```python
from build123d import *

# Parameters (mm, degrees)
SKETCH2_R           = 2.5
BOSS_EXTRUDE1_DEPTH = 12
CUT_EXTRUDE1_DEPTH  = 2.2
CHAMFER1_SIZE       = 0.55
CHAMFER2_SIZE       = 0.35
CHAMFER2_SIZE2      = 0.6


with BuildPart() as part:
    # Sketch1 → Revolve1 (revolve)
    with BuildSketch(Plane.XY.offset(9.9)):
        with BuildLine():
            Line((2.4, 14.65), (2.4, 9.9))
            Line((2.4, 9.9), (5.15, 9.9))
            Line((5.15, 9.9), (5.15, 11.8))
            ThreePointArc((5.15, 11.8), (4.281848259, 13.427774941), (2.899999999, 14.65))
            Line((2.899999999, 14.65), (2.4, 14.65))
        make_face()
    revolve(axis=Axis((2.4, 9.9, 9.9), (1, 0, 0)))

    # Sketch2 → Boss-Extrude1 (add)
    with BuildSketch(Plane.ZY.offset(-2.4)):
        with Locations((9.9, 9.9)):
            Circle(SKETCH2_R)
    extrude(amount=BOSS_EXTRUDE1_DEPTH)

    # Sketch3 → Cut-Extrude1 (cut)
    with BuildSketch(Plane(origin=(5.15, 0, 0), x_dir=(0, 0, -1), z_dir=(1, 0, 0))):
        Polygon((-11.6320508, 9.9), (-10.766025397, 8.400000002), (-9.033974587, 8.400000002), (-8.167949184, 9.9), (-9.033974587, 11.399999998), (-10.766025397, 11.399999998), align=None)
    extrude(amount=-CUT_EXTRUDE1_DEPTH, mode=Mode.SUBTRACT)

    # Chamfer1
    chamfer1_edges = [part.edges().sort_by_distance(p)[0] for p in [
        (-9.6, 9.9, 7.4),
    ]]
    chamfer(chamfer1_edges, length=CHAMFER1_SIZE)

    # Chamfer2
    chamfer2_edges = [part.edges().sort_by_distance(p)[0] for p in [
        (2.4, 9.9, 7.4),
    ]]
    chamfer2_side = [part.faces().sort_by_distance(p)[0] for p in [
        (2.4, 5.284350289, 9.9),
    ]]
    chamfer(chamfer2_edges, length=CHAMFER2_SIZE, length2=CHAMFER2_SIZE2, reference=chamfer2_side[0])


solid = part.part
```
Source: CAD feature listing. Evaluate the final solid. Frame: model axes, mm. A direction names the side the tool comes from. Give positions to 0.01 mm unless a question says otherwise; leave off trailing zeros. Loops run counter-clockwise (first coordinate to the right, second up) from the corner with the lowest first, then second, coordinate; pieces in that order, holes last. Notation, with made-up numbers: (6, 67.25) -> (46, 67.25) arc R12 cw to (46, 73.25) -> close; hole circle Ø10 at (36.25, 73). An arc over 180 degrees is marked (long way). Put each result on its own line as item: value. Start each with the question number.
1) Draft query along Z for faces 4 (the face through (2.4, 9.8, 6.8)), 5 (the face through (4, 8.4, 10)), 6 (the face through (2.646, 14.288, 8.081)). Return one class per face: released by +Z, released by -Z, zero draft, split by the parting line, or undercut.
2) Material intervals for probe 1 along X at (y, z) = (11, 10.5); probe 2 along Z at (x, y) = (3.75, 11.25); probe 3 along X at (y, z) = (14, 8.5), sorted ascending.
3) Cut plane A-A (x = -0.25). Return loops of the section in (y, z).
4) Contact query for flat-ended pins moving along their axis: P1, Ø4, axis at x = -1.5, y = 9, coming from the +Z side; P2, Ø5, axis at y = 10, z = 7.5, coming from the -X side; P3, Ø1.5, axis at y = 9.5, z = 9.5, coming from the +X side; P4, Ø1, axis at x = -5, z = 10.5, coming from the +Y side. Output: stop coordinate, or through.
5) Reachability of faces 1 (the face through (4.065, 10.66, 11.193)), 2 (the face through (-9.6, 10, 10)), 3 (the face through (-3.55, 11.59, 8.06)) from +Z, -Z, +X, -X, +Y, -Y: full face, straight path, thin tool, end or side. Return the list, or none.
6) Cut plane B-B (x = 2). Return loops of the section in (y, z).
Results are:
1. face 4: zero draft
1. face 5: undercut
1. face 6: split by the parting line
2. probe 1: x = -9.6 to 2.95
2. probe 2: z = 6.02 to 8.95, 10.85 to 13.78
2. probe 3: x = 2.4 to 3.49
3. outline: circle Ø5 at (9.9, 9.9)
4. P1: stops at z = 12.4
4. P2: stops at x = -9.6
4. P3: stops at x = 2.95
4. P4: stops at y = 12.4
5. face 1: +X
5. face 2: +Z, -Z, -X, +Y, -Y
5. face 3: -X
6. outline: circle Ø5.23 at (9.9, 9.9)
